Read the model definition and answer for the solid it produces. Units are mm, in the model's axes. A direction names the side the tool comes from. Coordinates: 2 decimals unless noted, no trailing zeros. Loops run counter-clockwise (first coordinate to the right, second up) from the corner with the lowest first, then second, coordinate; pieces in that order, holes last. Notation, with made-up numbers: (28, 46.5) -> (80, 46.5) arc R15 cw to (80, 75.5) -> close; hole circle Ø8 at (16, 37). An arc over 180 degrees is marked (long way). One line per question, with ' | ' between items. Start each with the question number.
```python
from build123d import *

# Parameters (mm, degrees)
BOSS_EXTRUDE1_DEPTH            = 1.6
BOSS_EXTRUDE2_DEPTH            = 0.1
M2_HOLE1_FIXINGSTRUCTURE_D     = 2.4
M2_HOLE1_FIXINGSTRUCTURE_DEPTH = 200
M2_HOLE1_FIXINGSTRUCTURE_TIP   = 0.721032743
SKETCH5_R                      = 1.1
CUT_EXTRUDE1_DEPTH             = 1.7


with BuildPart() as part:
    # Sketch1 → Boss-Extrude1 (new body)
    with BuildSketch(Plane.XY):
        with BuildLine():
            Line((-34, 44), (-34, 38))
            ThreePointArc((-34, 38), (-34.146446609, 37.646446609), (-34.5, 37.5))
            Line((-34.5, 37.5), (-40.5, 37.5))
            ThreePointArc((-40.5, 37.5), (-40.853553391, 37.353553391), (-41, 37))
            Line((-41, 37), (-41, -37))
            ThreePointArc((-41, -37), (-40.853553391, -37.353553391), (-40.5, -37.5))
            Line((-40.5, -37.5), (-34.5, -37.5))
            ThreePointArc((-34.5, -37.5), (-34.146446609, -37.646446609), (-34, -38))
            Line((-34, -38), (-34, -44))
            ThreePointArc((-34, -44), (-33.853553391, -44.353553391), (-33.5, -44.5))
            Line((-33.5, -44.5), (33.5, -44.5))
            ThreePointArc((33.5, -44.5), (33.853553391, -44.353553391), (34, -44))
            Line((34, -44), (34, -38))
            ThreePointArc((34, -38), (34.146446609, -37.646446609), (34.5, -37.5))
            Line((34.5, -37.5), (40.5, -37.5))
            ThreePointArc((40.5, -37.5), (40.853553391, -37.353553391), (41, -37))
            Line((41, -37), (41, 37))
            ThreePointArc((41, 37), (40.853553391, 37.353553391), (40.5, 37.5))
            Line((40.5, 37.5), (34.5, 37.5))
            ThreePointArc((34.5, 37.5), (34.146446609, 37.646446609), (34, 38))
            Line((34, 38), (34, 44))
            ThreePointArc((34, 44), (33.853553391, 44.353553391), (33.5, 44.5))
            Line((33.5, 44.5), (-33.5, 44.5))
            ThreePointArc((-33.5, 44.5), (-33.853553391, 44.353553391), (-34, 44))
        make_face()
    extrude(amount=BOSS_EXTRUDE1_DEPTH)

    # Esboço1 → Boss-Extrude2 (add)
    with BuildSketch(Plane.XY.offset(1.6)):
        with BuildLine():
            Line((-29.5, -37.5), (29.5, -37.5))
            ThreePointArc((29.5, -37.5), (33.035533906, -36.035533906), (34.5, -32.5))
            Line((34.5, -32.5), (34.5, 32.5))
            ThreePointArc((34.5, 32.5), (33.035533906, 36.035533906), (29.5, 37.5))
            Line((29.5, 37.5), (-29.5, 37.5))
            ThreePointArc((-29.5, 37.5), (-33.035533906, 36.035533906), (-34.5, 32.5))
            Line((-34.5, 32.5), (-34.5, -32.5))
            ThreePointArc((-34.5, -32.5), (-33.035533906, -36.035533906), (-29.5, -37.5))
        make_face()
    extrude(amount=BOSS_EXTRUDE2_DEPTH)

    # M2 Hole1-FixingStructure
    with Locations(Plane(origin=(0, 0, 0), x_dir=(-1, 0, 0), z_dir=(0, 0, -1))):
        with Locations((-30.5, 40.5), (30.5, 40.5), (-30.5, -40.5), (30.5, -40.5)):
            Hole(M2_HOLE1_FIXINGSTRUCTURE_D / 2, depth=M2_HOLE1_FIXINGSTRUCTURE_DEPTH)
            with Locations((0, 0, -(M2_HOLE1_FIXINGSTRUCTURE_DEPTH + M2_HOLE1_FIXINGSTRUCTURE_TIP / 2))):  # 118° drill point
                Cone(0, M2_HOLE1_FIXINGSTRUCTURE_D / 2, M2_HOLE1_FIXINGSTRUCTURE_TIP, mode=Mode.SUBTRACT)

    # Sketch5 → Cut-Extrude1 (cut)
    with BuildSketch(Plane.XY.offset(1.7)):
        with Locations((27.155444566, 3)):
            Circle(SKETCH5_R)
        with Locations((12, 29.25)):
            Circle(SKETCH5_R)
        with Locations((-3.155444566, 3)):
            Circle(SKETCH5_R)
    extrude(amount=-CUT_EXTRUDE1_DEPTH, mode=Mode.SUBTRACT)


solid = part.part
```
(1) Section A-A on z = 0.85 is taken. Give the number of separate pieces and of enclosed holes in the cut face, plus the area to 3 significant figures.
(2) Each of these flat-tipped pins is pushed along its axis until it touches: pin 1 Ø0.5 at (y, z) = (-41.5, 1) entering from -X; pin 2 Ø0.5 at (x, z) = (36, 1) entering from -Y; pin 3 Ø0.8 at (x, z) = (-38.5, 0.5) entering from +Y. Where does it stop, or does it pass through?
(3) Section D-D on y = 40.5 is taken. Write down the section's boundary in (x, z), plus the area to 3 significant figures.
(4) A tool of negligible diameter and unlimited length cuts with its end or side. For faces 3 (the cylindrical face through (-29.85, 41.51, 0.81)), 4 (the flat face through (-37, 0, 1.6)), from which of +Z, -Z, +X, -X, +Y, -Y can it reach the whole face along a straight path? Write none if from no direction.
(5) Section C-C on x = 12 is taken. Write down the section's boundary in (y, z), plus the area to 3 significant figures.
(6) Find the intervals of material crossed by probe 1 along Y at (x, z) = (30.5, 0.65); probe 2 along Y at (x, z) = (12, 0.5); probe 3 along X at (y, z) = (-39, 0.35), in increasing order. Write a range as from..to.
(7) Section B-B on y = 29.25 is taken. Write down the section's boundary in (x, z).
(8) Determine the mould class of faces 1 (the flat face through (-1, 1, 0)), 2 (the cylindrical face through (-2.106, 3.33, 0.862)) for opening direction Y: +Y half, -Y half, draft (parallel to the pull), parting line (faces both ways), or undercut.
Working result:
1) separate pieces: 1 | enclosed holes: 7 | area: 7,070 mm2
2) pin 1: stops at x = -34 | pin 2: stops at y = -37.5 | pin 3: stops at y = 37.5
3) outline: (-34, 0) -> (-31.7, 0) -> (-31.7, 1.6) -> (-34, 1.6) -> close; (-29.3, 0) -> (29.3, 0) -> (29.3, 1.6) -> (-29.3, 1.6) -> close; (31.7, 0) -> (34, 0) -> (34, 1.6) -> (31.7, 1.6) -> close | area: 101 mm2
4) face 3: +Z, -Z | face 4: +Z
5) outline: (-44.5, 0) -> (28.15, 0) -> (28.15, 1.7) -> (-37.5, 1.7) -> (-37.5, 1.6) -> (-44.5, 1.6) -> close; (30.35, 0) -> (44.5, 0) -> (44.5, 1.6) -> (37.5, 1.6) -> (37.5, 1.7) -> (30.35, 1.7) -> close | area: 146 mm2
6) probe 1: y = -44.5..-41.7, -39.3..39.3, 41.7..44.5 | probe 2: y = -44.5..28.15, 30.35..44.5 | probe 3: x = -34..34
7) outline: (-41, 0) -> (10.9, 0) -> (10.9, 1.7) -> (-34.5, 1.7) -> (-34.5, 1.6) -> (-41, 1.6) -> close; (13.1, 0) -> (41, 0) -> (41, 1.6) -> (34.5, 1.6) -> (34.5, 1.7) -> (13.1, 1.7) -> close
8) face 1: draft | face 2: undercut
